Geometry: see drawing. Coordinates: mm, zero at the bounding-box minimum. Coordinates: 2 decimals unless noted, no trailing zeros. Loops run counter-clockwise (first coordinate to the right, second up) from the corner with the lowest first, then second, coordinate; pieces in that order, holes last. Notation, with made-up numbers: (75, 61) - (97, 61) arc R20 ccw to (97, 66) - close; hole circle Ø7 at (86, 77.25). An arc over 180 degrees is marked (long way). Answer in a Markdown table with one row per item.
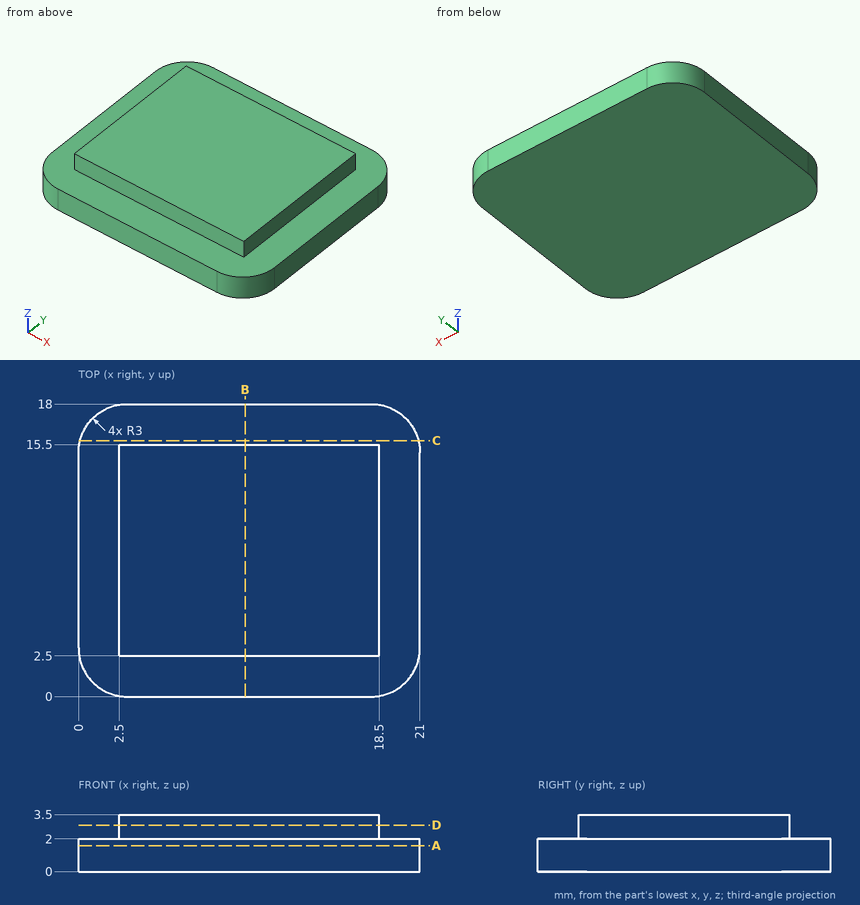
(1) First-contact query: pin 1 Ø1.2 at (x, z) = (11.5, 3) entering from +Y; pin 2 Ø1.2 at (x, z) = (7, 3) entering from -Y; pin 3 Ø2 at (y, z) = (2.5, 1.5) entering from -X; pin 4 Ø0.8 at (y, z) = (8.5, 3) entering from +X. Flat tips, straight axial feed; report the tip coordinate or a pass-through.
Verdict:
| item | result |
|---|---|
| pin 1 | stops at y = 15.5 |
| pin 2 | stops at y = 2.5 |
| pin 3 | stops at x = 0 |
| pin 4 | stops at x = 18.5 |
(2) Cut plane D-D on z = 2.85. Output: boundary loops of the cut face in (x, y), then the cut area to 3 significant figures.
Verdict:
| item | result |
|---|---|
| outline | (2.5, 2.5) - (18.5, 2.5) - (18.5, 15.5) - (2.5, 15.5) - close |
| area | 208 mm² |
(3) Cut plane C-C on y = 15.75. Output: boundary loops of the cut face in (x, z), then the cut area to 3 significant figures.
Verdict:
| item | result |
|---|---|
| outline | (0.1, 0) - (20.9, 0) - (20.9, 2) - (0.1, 2) - close |
| area | 41.6 mm² |
(4) Ray query, probe 1 along Z at (x, y) = (2, 4.5); probe 2 along Y at (x, z) = (6.5, 3.25); probe 3 along X at (y, z) = (10.75, 2.85). Return the intervals inside material, ascending.
Verdict:
| item | result |
|---|---|
| probe 1 | z = 0 to 2 |
| probe 2 | y = 2.5 to 15.5 |
| probe 3 | x = 2.5 to 18.5 |
(5) Cut plane A-A on z = 1.6. Output: boundary loops of the cut face in (x, y), then the cut area to 3 significant figures.
Verdict:
| item | result |
|---|---|
| outline | (0, 3) arc R3 ccw to (3, 0) - (18, 0) arc R3 ccw to (21, 3) - (21, 15) arc R3 ccw to (18, 18) - (3, 18) arc R3 ccw to (0, 15) - close |
| area | 370 mm² |
(6) Cut plane B-B on x = 10.25. Output: boundary loops of the cut face in (y, z), then the cut area to 3 significant figures.
Verdict:
| item | result |
|---|---|
| outline | (0, 0) - (18, 0) - (18, 2) - (15.5, 2) - (15.5, 3.5) - (2.5, 3.5) - (2.5, 2) - (0, 2) - close |
| area | 55.5 mm² |
